Build history of the part. All positions in model axes, mm. A direction names the side the tool comes from. Round coordinates to 2 decimals unless told otherwise and drop trailing zeros. Write each loop counter-clockwise with the first axis right and the second up, starting at its lowest first coordinate (ties: lowest second). Pieces come first, ordered by that corner, then holes. Notation, with made-up numbers: (49, -15.75) -> (106, -15.75) arc R25 cw to (106, -0.75) -> close; hole circle Ø7 at (33.25, 64.25). An arc over 180 degrees is marked (long way). Answer as CSV lines item,"result".
from build123d import *

# Parameters (mm, degrees)
SKETCH_R          = 5
PAD_DEPTH         = 5.5
SKETCH001_R       = 1.5
PAD001_DEPTH      = 3
PAD001_DEPTH_BACK = 8.5


with BuildPart() as part:
    # Sketch → Pad (new body)
    with BuildSketch(Plane.XY):
        Circle(SKETCH_R)
    extrude(amount=PAD_DEPTH)

    # Sketch001 → Pad001 (new body, two sides)
    with BuildSketch(Plane.XY.offset(5.5)) as pad001_sk:
        Circle(SKETCH001_R)
    extrude(amount=PAD001_DEPTH)
    extrude(pad001_sk.sketch, amount=-PAD001_DEPTH_BACK)


solid = part.part
1. Drop flat-ended pins along their axis: pin 1 Ø1 at (x, y) = (2, 3.5) entering from +Z; pin 2 Ø5 at (y, z) = (3, 0.5) entering from +X; pin 3 Ø1.5 at (y, z) = (0.5, 5) entering from -X; pin 4 Ø2 at (x, z) = (1.5, 0) entering from -Y. Give the stop position or say it passes through.
Results found:
pin 1,"stops at z = 5.5"
pin 2,"stops at x = 4.97"
pin 3,"stops at x = -5"
pin 4,"stops at y = -4.97"
2. Cut at D-D, the plane y = 3. Write the cut outline in (x, z).
Results found:
outline,"(-4, 0) -> (4, 0) -> (4, 5.5) -> (-4, 5.5) -> close"
3. Cut at C-C, the plane z = 1.25. Write the cut outline in (x, y).
Results found:
outline,"circle Ø10 at (0, 0)"
4. Cut at A-A, the plane y = 0. Write the cut outline in (x, z).
Results found:
outline,"(-5, 0) -> (-1.5, 0) -> (-1.5, -3) -> (1.5, -3) -> (1.5, 0) -> (5, 0) -> (5, 5.5) -> (1.5, 5.5) -> (1.5, 8.5) -> (-1.5, 8.5) -> (-1.5, 5.5) -> (-5, 5.5) -> close"
5. Probe line 1 along Y through (x, z) = (0, 5.75); line 2 along Z through (x, y) = (-2.5, -2.5); line 3 along Y through (x, z) = (-2.5, 2.5). List the from-to ranges inside material, lowest first.
Results found:
line 1,"y = -1.5 to 1.5"
line 2,"z = 0 to 5.5"
line 3,"y = -4.33 to 4.33"
6. Which spindle directions (+Z, -Z, +X, -X, +Y, -Y) get a long thin tool onto all of the face, cutting with end or side? Do faces 1 (the cylindrical face through (-1.5, 0.07, -1.48)), 2 (the cylindrical face through (-1.5, 0.07, 6.98)), 3 (the flat face through (0, 0, 8.5)). Say none if no direction does.
Results found:
face 1,"-Z"
face 2,"+Z"
face 3,"+Z, +X, -X, +Y, -Y"
